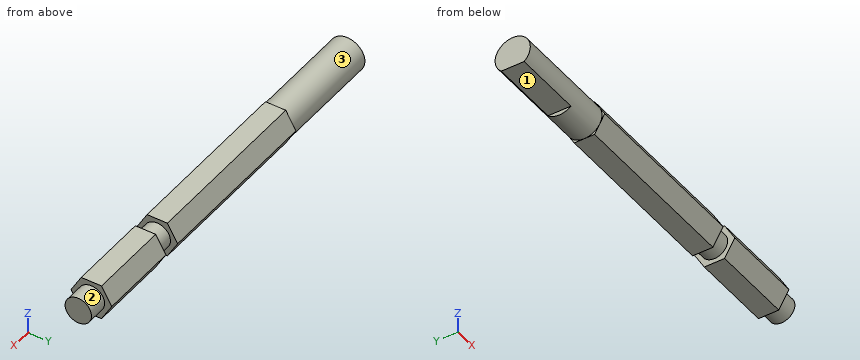
from build123d import *

# Parameters (mm, degrees)
SKETCH1_R               = 6.35
BOSS_EXTRUDE1_DEPTH     = 146.05
CUT_EXTRUDE1_DEPTH      = 1
CUT_EXTRUDE1_DEPTH_BACK = 25.4
BOSS_EXTRUDE2_START     = -7.112
BOSS_EXTRUDE2_DEPTH     = 100.0125
SKETCH5_R               = 6.35
SKETCH5_R_2             = 4.7625
CUT_EXTRUDE2_DEPTH      = 7.112
CUT_EXTRUDE3_START      = -36.5125
SKETCH6_R               = 19.82685814
SKETCH6_R_2             = 4.7625
CUT_EXTRUDE3_DEPTH      = 6.35


with BuildPart() as part:
    # Sketch1 → Boss-Extrude1 (new body)
    with BuildSketch(Plane(origin=(0, 0, 0), x_dir=(0, 0, -1), z_dir=(1, 0, 0))):
        Circle(SKETCH1_R)
    extrude(amount=BOSS_EXTRUDE1_DEPTH)

    # Sketch2 → Cut-Extrude1 (cut, two sides)
    with BuildSketch(Plane.ZY) as cut_extrude1_sk:
        Polygon((-4.826, -44.764945263), (-4.826, -4.12701151), (-4.826, 4.12701151), (-4.826, 44.764945263), (-86.101867507, 44.764945263), (-86.101867507, -44.764945263), align=None)
    extrude(amount=CUT_EXTRUDE1_DEPTH, mode=Mode.SUBTRACT)
    extrude(cut_extrude1_sk.sketch, amount=-CUT_EXTRUDE1_DEPTH_BACK, mode=Mode.SUBTRACT)

    # Sketch4 → Boss-Extrude2 (add)
    with BuildSketch(Plane(origin=(146.05, 0, 0), x_dir=(0, 0, -1), z_dir=(1, 0, 0)).offset(BOSS_EXTRUDE2_START)):
        Polygon((6.35, -3.666174209), (6.35, 3.666174209), (0, 7.332348419), (-6.35, 3.666174209), (-6.35, -3.666174209), (0, -7.332348419), align=None)
    extrude(amount=-BOSS_EXTRUDE2_DEPTH)

    # Sketch5 → Cut-Extrude2 (cut)
    with BuildSketch(Plane(origin=(146.05, 0, 0), x_dir=(0, 0, -1), z_dir=(1, 0, 0))):
        Circle(SKETCH5_R)
        Circle(SKETCH5_R_2, mode=Mode.SUBTRACT)
    extrude(amount=-CUT_EXTRUDE2_DEPTH, mode=Mode.SUBTRACT)

    # Sketch6 → Cut-Extrude3 (cut)
    with BuildSketch(Plane(origin=(146.05, 0, 0), x_dir=(0, 0, -1), z_dir=(1, 0, 0)).offset(CUT_EXTRUDE3_START)):
        Circle(SKETCH6_R)
        Circle(SKETCH6_R_2, mode=Mode.SUBTRACT)
    extrude(amount=-CUT_EXTRUDE3_DEPTH, mode=Mode.SUBTRACT)


solid = part.part
Work out the finished part from the listing and answer in its coordinate system (mm). Face numbers are marked on the shaded views. A direction names the side the tool comes from. Give positions to 0.01 mm unless a question says otherwise; leave off trailing zeros. Loops run counter-clockwise (first coordinate to the right, second up) from the corner with the lowest first, then second, coordinate; pieces in that order, holes last. Notation, with made-up numbers: (-29, 30.25) -> (-25, 30.25) arc R35 cw to (-25, 66.25) -> close; hole circle Ø1 at (46.25, -35.75). An arc over 180 degrees is marked (long way). Use a Markdown table: item, result. Add a question column.
1) Each of these flat-tipped pins is pushed along its axis until it touches: P1, Ø1, axis at x = 108, z = 4, coming from the -Y side; P2, Ø1.2, axis at y = -1.5, z = -5.5, coming from the -X side; P3, Ø4, axis at x = 11.5, y = -1, coming from the -Z side. Where does it stop, or does it pass through?
2) Consider line 1 along X through (y, z) = (2.5, -4.75); line 2 along Z through (x, y) = (33, 5.5); line 3 along Y through (x, z) = (58.5, 1.75). Determine where each line is inside the solid, lowest interval first.
3) Which of the six approach directions +Z, -Z, +X, -X, +Y, -Y give full straight-line access (tool end or side, diameter ignored) to the marked faces 1, 2 and 3?
4) The part is cut by section A-A, the plane x = 91.5. Determine the outline of the cut face in (y, z), plus the area to 3 significant figures.
5) The part is cut by section B-B, the plane x = 18. Determine the outline of the cut face in (y, z), plus the area to 3 significant figures.
Reported:
| question | item | result |
|---|---|---|
| 1 | P1 | stops at y = -3.23 |
| 1 | P2 | stops at x = 25.4 |
| 1 | P3 | stops at z = -4.83 |
| 2 | line 1 | x = 0 to 103.19, 109.54 to 138.94 |
| 2 | line 2 | z = -3.17 to 3.17 |
| 2 | line 3 | y = -6.32 to 6.32 |
| 3 | face 1 | -Z, -X, +Y, -Y |
| 3 | face 2 | +X |
| 3 | face 3 | -X |
| 4 | outline | (-7.33, 0) -> (-3.67, -6.35) -> (3.67, -6.35) -> (7.33, 0) -> (3.67, 6.35) -> (-3.67, 6.35) -> close |
| 4 | area | 140 mm^2 |
| 5 | outline | (-4.13, -4.83) -> (4.13, -4.83) arc R6.35 ccw (long way) to start |
| 5 | area | 118 mm^2 |
